Work out the finished part from the listing and answer in its coordinate system (mm). Round coordinates to 2 decimals unless told otherwise and drop trailing zeros. Write each loop counter-clockwise with the first axis right and the second up, starting at its lowest first coordinate (ties: lowest second). Pieces come first, ordered by that corner, then holes. Notation, with made-up numbers: M 33.5,71.25 L 83.5,71.25 A29 cw 83.5,109.25 Z; hole C 65.5,88 d9. An arc over 180 degrees is marked long. One line per item, written item: value. Start each with the question number.
Q1. Given pin 1 Ø3 at (y, z) = (4, 33.5) entering from -X; pin 2 Ø1.5 at (y, z) = (0.5, 17) entering from +X; pin 3 Ø1 at (x, z) = (1, 31) entering from -Y, each flat-ended and moving along its own axis, determine where each tip first touches the part or whether it passes through.
Q2. Consider probe 1 along X at (y, z) = (0.25, 29.5); probe 2 along Y at (x, z) = (0.25, 3); probe 3 along Y at (x, z) = (-2.25, 22.5). Determine where each line is inside the solid, lowest interval first.
Q3. Find section A-A (z = 21). Write down the section's boundary in (x, y).
Q4. The mould has two halves that part along Z. Classify faces 1 (the cylindrical face through (-0.69, 3.1, 8.47)), 2 (the cylindrical face through (-0.33, -2.52, 19.97)), 3 (the flat face through (0, 0, 41.275)), 4 (the conical face through (4.807, 1.514, 29.183)): released by +Z, released by -Z, zero draft, split by the parting line, or undercut.
Autodesk Inventor part; units mm, degrees
ref_plane "YZ Plane" through (0, 0, 0) normal (1, 0, 0) x (0, 1, 0)
ref_plane "XZ Plane" through (0, 0, 0) normal (0, 1, 0) x (-1, 0, 0)
ref_plane "XY Plane" through (0, 0, 0) normal (0, 0, 1) x (1, 0, 0)
sketch "Sketch1" plane through (0, 0, 0) normal (0, 0, 1) x (1, 0, 0)
  circle A0 centre (0, 0) radius 3.175
  dimension "d0" = 6.35
extrude "Extrusion1" add sketch "Sketch1" along normal blind 15.875
thread "Thread1"
chamfer "Chamfer1" distance 1.27 angle 45 1 edges at (-3.175, 0, 0)
sketch "Sketch3" plane through (0, 0, 15.875) normal (0, 0, 1) x (1, 0, 0)
  circle A0 centre (0, 0) radius 2.54
  dimension "d11" = 5.08
extrude "Extrusion3" add sketch "Sketch3" along normal blind 6.35
sketch "Sketch4" plane through (0, 0, 22.225) normal (0, 0, 1) x (1, 0, 0)
  circle A0 centre (0, 0) radius 3.175
  dimension "d14" = 6.35
extrude "Extrusion4" add sketch "Sketch4" along normal blind 19.05 draft 15
fillet "Fillet2" radius 3.175 3 edges at (-8.2794, 0, 41.275) (-3.175, 0, 22.225) (-2.54, 0, 15.875)
properties part number "peg"
The answers:
1. pin 1: x = -5.8
1. pin 2: x = 2.9
1. pin 3: y = -5.59
2. probe 1: -5.12 to 5.12
2. probe 2: -3.17 to 3.17
2. probe 3: -1.73 to 1.73
3. outline: C 0,0 d5.08
4. face 1: zero draft
4. face 2: undercut
4. face 3: released by +Z
4. face 4: released by -Z
